Input: part model. Units: mm. Frame: model coordinates. Face numbers are marked on the shaded views. Round coordinates to 2 decimals unless told otherwise and drop trailing zeros. Write each loop counter-clockwise with the first axis right and the second up, starting at its lowest first coordinate (ties: lowest second). Pieces come first, ordered by that corner, then holes. Notation, with made-up numbers: (85, -39) -> (114, -39) arc R19 cw to (114, -22) -> close; hole circle Ø4 at (31.5, -3.75). An arc over 180 degrees is marked (long way). Write item = value, one per line.
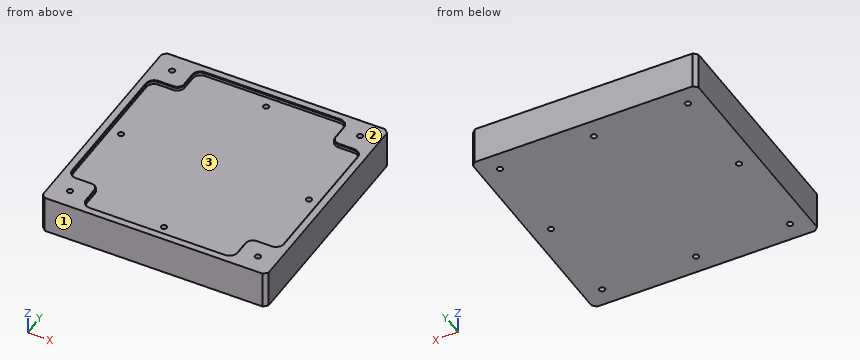
Autodesk Inventor part; units mm, degrees
ref_plane "YZ Plane" through (0, 0, 0) normal (1, 0, 0) x (0, 1, 0)
ref_plane "XZ Plane" through (0, 0, 0) normal (0, 1, 0) x (-1, 0, 0)
ref_plane "XY Plane" through (0, 0, 0) normal (0, 0, 1) x (1, 0, 0)
sketch "Sketch1" plane through (0, 0, 0) normal (0, 0, 1) x (1, 0, 0)
  line L0 (-150, -150) -> (150, -150)
  line L1 (150, -150) -> (150, 150)
  line L2 (150, 150) -> (-150, 150)
  line L3 (-150, 150) -> (-150, -150)
  line L4 (-150, -150) -> (150, 150) construction
  line L5 (150, -150) -> (-150, 150) construction
  point P0 (0, 0)
  dimension "d0" = 300
  dimension "d1" = 300
extrude "Extrusion1" add sketch "Sketch1" along normal blind 50
chamfer "Chamfer1" distance 5 angle 45 4 edges at (150, -150, 25) (150, 150, 25) (-150, 150, 25) (-150, -150, 25)
sketch "Sketch2" plane through (0, 0, 50) normal (0, 0, 1) x (1, 0, 0)
  line L0 (125, 194.8236) -> (125, -186.7434) construction
  line L1 (150, -145) -> (150, 145) construction
  line L2 (185.8456, 125) -> (-170.134, 125) construction
  line L3 (145, 150) -> (-145, 150) construction
  circle A0 centre (125, 125) radius 3.75
  circle A1 centre (125, 0) radius 3.75
  line L4 (-241.3299, 0) -> (257.0415, 0) construction
  line L5 (0, -263.0568) -> (0, 271.137) construction
  circle A2 centre (0, 125) radius 3.75
  circle A3 centre (125, -125) radius 3.75
  circle A4 centre (0, -125) radius 3.75
  line L6 (-150, -145) -> (-150, 145) construction
  circle A5 centre (-125, 125) radius 3.75
  circle A6 centre (-125, 0) radius 3.75
  circle A7 centre (-125, -125) radius 3.75
  point P0 (0, 0)
  point P1 (145, -150)
  point P2 (-125, 194.8236)
  point P3 (-185.8456, 125)
  point P4 (-145, -150)
  dimension "d7" = 25
  dimension "d8" = 125
  dimension "d9" = 25
  dimension "d10" = 7.5
  dimension "d11" = 7.5
  dimension "d12" = 7.5
extrude "Extrusion2" cut sketch "Sketch2" against normal through all
sketch "Sketch3" plane through (0, 0, 50) normal (0, 0, 1) x (1, 0, 0)
  line L0 (-100, 140) -> (100, 140)
  line L1 (100, 140) -> (100, -140)
  line L2 (100, -140) -> (-100, -140)
  line L3 (-100, -140) -> (-100, 140)
  line L4 (-100, 140) -> (100, -140) construction
  line L5 (100, 140) -> (-100, -140) construction
  line L6 (-140, 100) -> (140, 100)
  line L7 (140, 100) -> (140, -100)
  line L8 (140, -100) -> (-140, -100)
  line L9 (-140, -100) -> (-140, 100)
  line L10 (-140, 100) -> (140, -100) construction
  line L11 (140, 100) -> (-140, -100) construction
  line L12 (150, -145) -> (150, 145)
  line L13 (145, 150) -> (-145, 150)
  line L14 (-145, -150) -> (145, -150)
  point P0 (0, 0)
  point P1 (100, 100)
  point P2 (-100, 100)
  point P3 (-100, -100)
  point P4 (100, -100)
  dimension "d15" = 10
  dimension "d16" = 10
  dimension "d17" = 50
  dimension "d18" = 50
extrude "Extrusion3" cut sketch "Sketch3" against normal blind 5
fillet "Fillet1" radius 10 12 edges at (-100, 100, 47.5) (-100, -100, 47.5) (100, -100, 47.5) (100, 100, 47.5) (140, 100, 47.5) (140, -100, 47.5) (100, -140, 47.5) (-100, -140, 47.5) (-140, -100, 47.5) (-140, 100, 47.5) (-100, 140, 47.5) (100, 140, 47.5)
chamfer "Chamfer2" distance 1 angle 45 24 edges at (100, 120, 50) (102.9289, 102.9289, 50) (120, 100, 50) (137.0711, 97.0711, 50) (140, 0, 50) (137.0711, -97.0711, 50) (120, -100, 50) (102.9289, -102.9289, 50) (100, -120, 50) (97.0711, -137.0711, 50) (0, -140, 50) (-97.0711, -137.0711, 50) (-100, -120, 50) (-102.9289, -102.9289, 50) (-120, -100, 50) (-137.0711, -97.0711, 50) (-140, 0, 50) (-137.0711, 97.0711, 50) (-120, 100, 50) (-102.9289, 102.9289, 50) (-100, 120, 50) (-97.0711, 137.0711, 50) (0, 140, 50) (97.0711, 137.0711, 50)
equation "\"d1\" = d0"
equation "\"d9\" = d7"
equation "\"d11\" = d10"
equation "\"d12\" = d10"
equation "\"d18\" = d17"
properties part number "MDF_Block"
1) Cut plane B-B (x = 0). Return the cut outline in (y, z), and give its area (3 significant figures).
Solutions:
outline = (-150, 0) -> (-128.75, 0) -> (-128.75, 45) -> (-140, 45) -> (-140, 49) -> (-141, 50) -> (-150, 50) -> close; (-121.25, 0) -> (121.25, 0) -> (121.25, 45) -> (-121.25, 45) -> close; (128.75, 0) -> (150, 0) -> (150, 50) -> (141, 50) -> (140, 49) -> (140, 45) -> (128.75, 45) -> close
area = 12,900 mm^2
2) Line query: L1, parallel to Y at x = 125, z = 20.5; L2, parallel to Y at x = 0, z = 24; L3, parallel to Z at x = 111, y = -27. Output: solid intervals per line, ascending. Write a range as from..to.
Solutions:
L1 = -150..-128.75, -121.25..-3.75, 3.75..121.25, 128.75..150
L2 = -150..-128.75, -121.25..121.25, 128.75..150
L3 = 0..45
3) First-contact query: P1, Ø8.5, axis at x = 0, y = -125, coming from the +Z side; P2, Ø4.5, axis at x = 125, y = 125, coming from the +Z side. Flat tips, straight axial feed; report the tip coordinate or a pass-through.
Solutions:
P1 = 45
P2 = through
4) Cut plane A-A (y = 125). Return the cut outline in (x, z).
Solutions:
outline = (-150, 0) -> (-128.75, 0) -> (-128.75, 50) -> (-150, 50) -> close; (-121.25, 0) -> (-3.75, 0) -> (-3.75, 45) -> (-100, 45) -> (-100, 49) -> (-101, 50) -> (-121.25, 50) -> close; (3.75, 0) -> (121.25, 0) -> (121.25, 50) -> (101, 50) -> (100, 49) -> (100, 45) -> (3.75, 45) -> close; (128.75, 0) -> (150, 0) -> (150, 50) -> (128.75, 50) -> close
5) Cut plane D-D (y = -116). Return the cut outline in (x, z), and give its area (3 significant figures).
Solutions:
outline = (-150, 0) -> (150, 0) -> (150, 50) -> (101, 50) -> (100, 49) -> (100, 45) -> (-100, 45) -> (-100, 49) -> (-101, 50) -> (-150, 50) -> close
area = 14,000 mm^2
6) Draft query along Y for the marked faces 1, 2 and 3. Return one class per face: +Y half, -Y half, draft (parallel to the pull), parting line (faces both ways), or undercut.
Solutions:
face_1 = -Y half
face_2 = draft
face_3 = undercut
